Geometry: final body of the model. Coordinates: model frame, mm. Face numbers are marked on the shaded views. A direction names the side the tool comes from. Coordinates: 2 decimals unless noted, no trailing zeros. Order: outer loops, then holes, each group sorted by start corner. A loop starts at its lowest first (then second) coordinate and runs counter-clockwise, first axis right, second up. Notation, with made-up numbers: (77.5, 14) - (115.5, 14) arc R24 ccw to (115.5, 41) - close; hole circle Ø7 at (-35, -30.5). An arc over 180 degrees is marked (long way). Use a Markdown table: item, result. Add a question column.
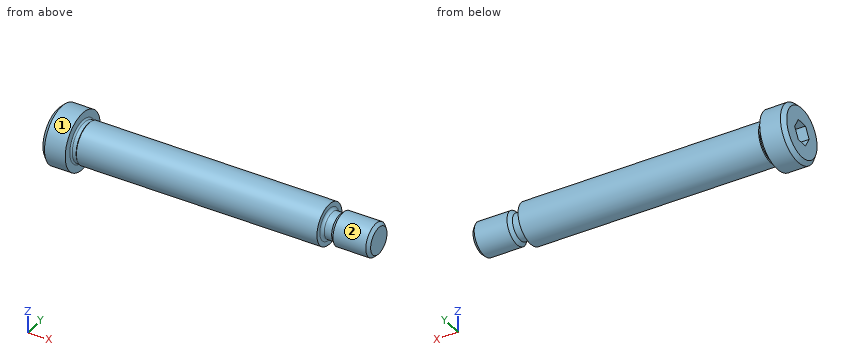
```python
from build123d import *

# Parameters (mm, degrees)
HEX_2_DEPTH = 5.9436


# Read off the part's stored shape, not the designer's step: ThreadSchematic
with BuildPart() as part:
    # ThreadSchematic outline → ThreadSchematic (revolve)
    with BuildSketch(Plane.YX):
        with BuildLine():
            Line((0, 123.825), (0, 0))
            Line((0, 0), (9.5885, 0))
            Line((9.5885, 0), (11.1125, 1.524))
            Line((11.1125, 1.524), (11.1125, 9.525))
            Line((11.1125, 9.525), (8.255, 9.525))
            ThreePointArc((8.255, 9.525), (7.823947706, 9.703547706), (7.6454, 10.1346))
            Line((7.6454, 10.1346), (7.6454, 11.6205))
            Line((7.6454, 11.6205), (7.9121, 11.8872))
            Line((7.9121, 11.8872), (7.9121, 104.775))
            Line((7.9121, 104.775), (6.1087, 104.775))
            ThreePointArc((6.1087, 104.775), (5.354358486, 105.087458486), (5.0419, 105.8418))
            Line((5.0419, 105.8418), (5.0419, 108.6866))
            Line((5.0419, 108.6866), (6.35, 109.9947))
            Line((6.35, 109.9947), (6.35, 122.66168))
            Line((6.35, 122.66168), (5.18668, 123.825))
            Line((5.18668, 123.825), (0, 123.825))
        make_face()
    revolve(axis=Axis((0, 0, 0), (1, 0, 0)))

    # Sketch2 → PreBroach (revolve, cut)
    with BuildSketch(Plane.XY, mode=Mode.PRIVATE) as prebroach_sk:
        Polygon((0, 3.9624), (5.9436, 3.9624), (8.231292707, 0), (0, 0), align=None)
    revolve(prebroach_sk.sketch.rotate(Axis((0, 0, 0), (1, 0, 0)), 90), axis=Axis((0, 0, 0), (1, 0, 0)), mode=Mode.SUBTRACT)

    # Sketch3 → Hex 2 (cut)
    with BuildSketch(Plane.ZY):
        Polygon((-3.9624, -2.287692707), (-3.9624, 2.287692707), (0, 4.575385413), (3.9624, 2.287692707), (3.9624, -2.287692707), (0, -4.575385413), align=None)
    extrude(amount=-HEX_2_DEPTH, mode=Mode.SUBTRACT)


solid = part.part
```
1) Ray query, line 1 along Y through (x, z) = (79.5, 2); line 2 along X through (y, z) = (-4.25, 7.25) (3 decimals); line 3 along Z through (x, y) = (48, 0.5). Return the intervals inside material, ascending.
2) Section A-A (x = 59). Return loops of the section in (y, z), then the cut area to 3 significant figures.
3) Set-up query: the marked faces 1 and 2. Return all of +Z, -Z, +X, -X, +Y, -Y with unobstructed straight access to the full face (end or side cutting, diameter ignored); none if empty.
4) Pin query (flat end, axial travel): pin 1 (6 mm diameter, centred on x = 70.5, z = 1, fed in from +Y); pin 2 (2 mm diameter, centred on x = 47, y = 1, fed in from +Z); pin 3 (0.9 mm diameter, centred on y = 4, z = -0.5, fed in from -X); pin 4 (12 mm diameter, centred on x = 27.5, z = -1.5, fed in from -Y). Return the tip coordinate at first contact, or that it passes through.
Values follow:
| question | item | result |
|---|---|---|
| 1 | line 1 | y = -7.66 to 7.66 |
| 1 | line 2 | x = 0 to 9.525 |
| 1 | line 3 | z = -7.9 to 7.9 |
| 2 | outline | circle Ø15.82 at (0, 0) |
| 2 | area | 197 mm² |
| 3 | face 1 | +X, -X |
| 3 | face 2 | +X |
| 4 | pin 1 | stops at y = 7.91 |
| 4 | pin 2 | stops at z = 7.91 |
| 4 | pin 3 | stops at x = 0 |
| 4 | pin 4 | stops at y = -7.91 |
